Print and shaded views of the part. All mm, measured from the part's lowest x, y and z. Round coordinates to 2 decimals unless told otherwise and drop trailing zeros. Write each loop counter-clockwise with the first axis right and the second up, starting at its lowest first coordinate (ties: lowest second). Pieces come first, ordered by that corner, then holes.
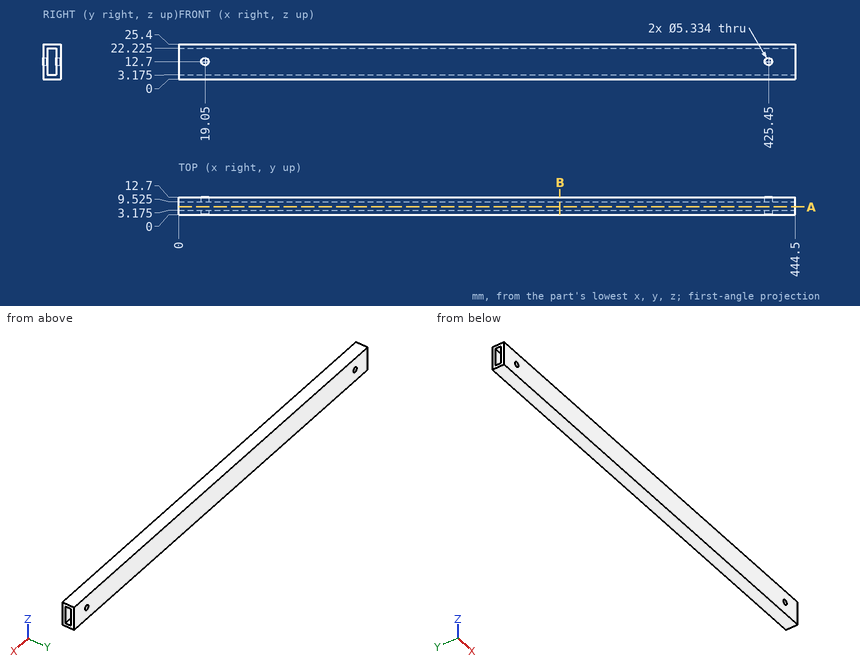
1) Slice it at A-A (y = 5.75). Write the cut outline in (x, z) (3 decimals), plus the area to 3 significant figures.
Results:
outline: (0, 0) - (444.5, 0) - (444.5, 3.175) - (0, 3.175) - close; (0, 22.225) - (444.5, 22.225) - (444.5, 25.4) - (0, 25.4) - close
area: 2,820 mm2
2) Pin check, flat tip, straight feed: pin 1 Ø4.5 at (x, z) = (19.05, 12.7) entering from -Y (3 decimals). Stop position of the tip, or through.
Results:
pin 1: passes through
3) Wall check: L1, parallel to X at y = 1.5, z = 12.7; L2, parallel to Z at x = 372, y = 4.75 (3 decimals); L3, parallel to Y at x = 179.5, z = 16.75 (3 decimals). Give the ranges that are in metal, low to high.
Results:
L1: x = 0 to 16.38, 21.72 to 422.78, 428.12 to 444.5
L2: z = 0 to 3.175, 22.225 to 25.4
L3: y = 0 to 3.175, 9.525 to 12.7
4) Slice it at B-B (x = 275). Write the cut outline in (y, z) (3 decimals), plus the area to 3 significant figures.
Results:
outline: (0, 0) - (12.7, 0) - (12.7, 25.4) - (0, 25.4) - close; hole (3.175, 3.175) - (9.525, 3.175) - (9.525, 22.225) - (3.175, 22.225) - close
area: 202 mm2
